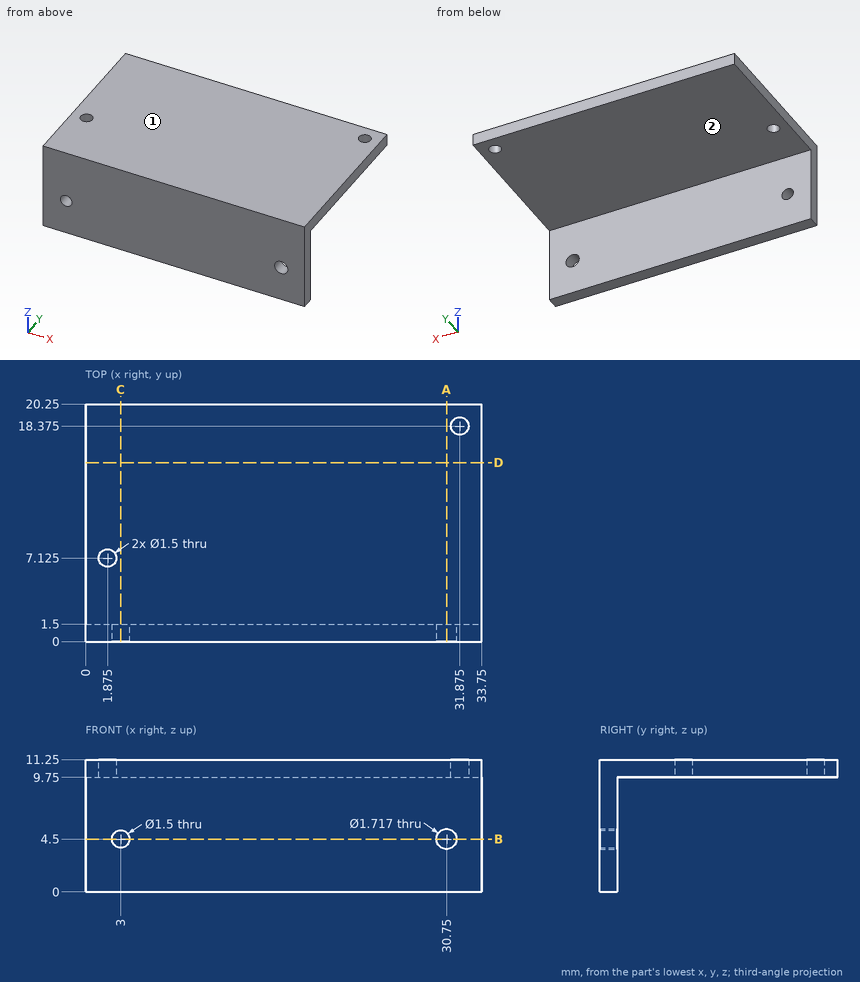
Geometry check sheet. Reference: drawing and pictorial views, mm from the part's lowest x, y, z. A direction names the side the tool comes from. Coordinates: 2 decimals unless noted, no trailing zeros. Loops run counter-clockwise (first coordinate to the right, second up) from the corner with the lowest first, then second, coordinate; pieces in that order, holes last. Notation, with made-up numbers: (13.25, -33.75) - (24.25, -33.75) arc R14 ccw to (24.25, -13.75) - close; hole circle Ø2 at (48, -27). An arc over 180 degrees is marked (long way). Return JSON: item names as keys, results as strings.
1. Tool access check on the marked faces 1 and 2. Record the directions out of +Z, -Z, +X, -X, +Y, -Y that give a thin tool (end or side, any length) a straight path to the whole face; none if there is none.
Established:
{"face 1": "+Z, +X, -X, +Y, -Y", "face 2": "-Z, +X, -X, +Y"}
2. Thickness scan on L1, parallel to Z at x = 3, y = 1.1; L2, parallel to Z at x = 24.5, y = 17.75; L3, parallel to Z at x = 30.75, y = 0.7. Record the ranges inside material, lowest first.
Established:
{"L1": "z = 0 to 3.75, 5.25 to 11.25", "L2": "z = 9.75 to 11.25", "L3": "z = 0 to 3.64, 5.36 to 11.25"}
3. Section check B-B, the plane z = 4.5. Record the boundary of the cut face in (x, y), then the cut area to 3 significant figures.
Established:
{"outline": "(0, 0) - (2.25, 0) - (2.25, 1.5) - (0, 1.5) - close; (3.75, 0) - (29.89, 0) - (29.89, 1.5) - (3.75, 1.5) - close; (31.61, 0) - (33.75, 0) - (33.75, 1.5) - (31.61, 1.5) - close", "area": "45.8 mm2"}
4. Section check D-D, the plane y = 15.25. Record the boundary of the cut face in (x, z).
Established:
{"outline": "(0, 9.75) - (33.75, 9.75) - (33.75, 11.25) - (0, 11.25) - close"}
5. Section check A-A, the plane x = 30.75. Record the boundary of the cut face in (y, z).
Established:
{"outline": "(0, 0) - (1.5, 0) - (1.5, 3.64) - (0, 3.64) - close; (0, 5.36) - (1.5, 5.36) - (1.5, 9.75) - (20.25, 9.75) - (20.25, 11.25) - (0, 11.25) - close"}
6. Section check C-C, the plane x = 3. Record the boundary of the cut face in (y, z).
Established:
{"outline": "(0, 0) - (1.5, 0) - (1.5, 3.75) - (0, 3.75) - close; (0, 5.25) - (1.5, 5.25) - (1.5, 9.75) - (20.25, 9.75) - (20.25, 11.25) - (0, 11.25) - close"}
7. Go/stop test with flat-tipped pins: pin 1 (2 mm diameter, centred on y = 15.5, z = 10, fed in from -X); pin 2 (1 mm diameter, centred on x = 4.5, y = 8.5, fed in from -Z); pin 3 (3 mm diameter, centred on x = 19, z = 2.5, fed in from +Y). Record where each tip stops, or that it passes through.
Established:
{"pin 1": "stops at x = 0", "pin 2": "stops at z = 9.75", "pin 3": "stops at y = 1.5"}
